For this review, take the finished solid that the model builds, in its own axes (mm). A direction names the side the tool comes from. Round coordinates to 2 decimals unless told otherwise and drop trailing zeros. Write each loop counter-clockwise with the first axis right and the second up, starting at its lowest first coordinate (ties: lowest second). Pieces come first, ordered by that corner, then holes. Notation, with made-up numbers: M 29.5,31 L 67.5,31 A30 ccw 67.5,63 Z; hole C 2,77.5 d11. An arc over 180 degrees is marked long. Use one line per item in the form item = value. Start each with the question number.
Item 1: Add section B-B (y = -8.25). State the section outline as (x, z) points.
Item 2: For faces 4 (the cylindrical face through (-19.274, 5.334, -19.435)), 5 (the flat face through (0, 0, 0)), list the 3-axis set-ups (+Z, -Z, +X, -X, +Y, -Y) from which the entire face can be reached by the end or side of a thin tool; tool diameter is ignored.
Item 3: For line 1 (Z direction, x = 17.5, y = 6.25) (3 decimals); line 2 (X direction, y = 6.25, z = -17.5) (3 decimals); line 3 (X direction, y = -8.25, z = -13), list the stretches that pass through material, from the lowest coordinate up. Write a range as [from, to].
Item 4: Add section A-A (z = 17.5). State the section outline as (x, y) points (3 decimals), and give its area (3 significant figures).
Item 5: Add section C-C (x = -17.5). State the section outline as (y, z) points (3 decimals), and give its area (3 significant figures).
Item 6: Draft analysis for pull direction Z (two halves, no side actions). For faces 1 (the flat face through (26, -12, 0)), 2 (the flat face through (0, 4, -25)), 3 (the cylindrical face through (15.726, 5.334, -19.435)), state which applies: released by +Z, released by -Z, zero draft, split by the parting line, or undercut.
Item 7: Add section D-D (y = 7.25). State the section outline as (x, z) points (3 decimals).
Item 8: For P1, Ø3, axis at x = -15.5, z = -2, coming from the -Y side, flat-tipped, find the tip position at first contact; note if it passes through.
Autodesk Inventor part; units mm, degrees
ref_plane "YZ Plane" through (0, 0, 0) normal (1, 0, 0) x (0, 1, 0)
ref_plane "XZ Plane" through (0, 0, 0) normal (0, 1, 0) x (-1, 0, 0)
ref_plane "XY Plane" through (0, 0, 0) normal (0, 0, 1) x (1, 0, 0)
sketch "Sketch1" plane through (0, 0, 0) normal (0, 1, 0) x (-1, 0, 0)
  line L0 (29, -25) -> (-29, -25)
  line L1 (-29, -25) -> (-29, 25)
  line L2 (-29, 25) -> (29, 25)
  line L3 (29, 25) -> (29, -25)
  line L4 (29, -25) -> (-29, 25) construction
  line L5 (-29, -25) -> (29, 25) construction
  point P0 (0, 0)
  dimension "d0" = 58
  dimension "d1" = 50
extrude "Extrusion1" add sketch "Sketch1" along normal blind 10.8204
sketch "Sketch2" plane through (0, 0, 0) normal (0, -1, 0) x (1, 0, 0)
  line L0 (-29, -25) -> (29, -25)
  line L1 (29, -25) -> (29, 25)
  line L2 (29, 25) -> (-29, 25)
  line L3 (-29, 25) -> (-29, -25)
  line L4 (-24, 25) -> (-24, -25)
  line L5 (24, 25) -> (24, -25)
  point P0 (0, 0)
  dimension "d4" = 5
  dimension "d5" = 5
extrude "Extrusion2" add sketch "Sketch2" along normal blind 12 contours L3 L2 L4 L0 | L5 L2 L1 L0
sketch "Sketch3" plane through (0, 10.8204, 0) normal (0, 1, 0) x (1, 0, 0)
  line L0 (29, 25) -> (-29, 25)
  line L1 (-29, 25) -> (-29, -25)
  point P0 (0, 0)
  point P1 (-17.5, 17.5)
  point P2 (17.5, 17.5)
  point P3 (-17.5, -17.5)
  point P4 (17.5, -17.5)
  dimension "d10" = 35
  dimension "d13" = 35
  dimension "d16" = 11.5
  dimension "d17" = 58
  dimension "d18" = 50
  dimension "d19" = 7.5
hole "Hole1" at (-17.5, 10.8204, -17.5) at (17.5, 10.8204, -17.5) at (-17.5, 10.8204, 17.5) at (17.5, 10.8204, 17.5) direction (0, -1, 0) diameter 5.25 end through all
equation "\"d5\" = d4"
properties part number "sbr20uu_standoff"
Calculated:
q1.outline = M -29,-25 L -24,-25 L -24,25 L -29,25 Z; M 24,-25 L 29,-25 L 29,25 L 24,25 Z
q2.face_4 = +Y, -Y
q2.face_5 = +Z, -Z, -Y
q3.line_1 = [-25, -20.125], [-14.875, 14.875], [20.125, 25]
q3.line_2 = [-29, -20.125], [-14.875, 14.875], [20.125, 29]
q3.line_3 = [-29, -24], [24, 29]
q4.outline = M -29,-12 L -24,-12 L -24,0 L -20.125,0 L -20.125,10.82 L -29,10.82 Z; M -14.875,0 L 14.875,0 L 14.875,10.82 L -14.875,10.82 Z; M 20.125,0 L 24,0 L 24,-12 L 29,-12 L 29,10.82 L 20.125,10.82 Z
q4.area = 634 mm^2
q5.outline = M 0,-25 L 10.82,-25 L 10.82,-20.125 L 0,-20.125 Z; M 0,-14.875 L 10.82,-14.875 L 10.82,14.875 L 0,14.875 Z; M 0,20.125 L 10.82,20.125 L 10.82,25 L 0,25 Z
q5.area = 427 mm^2
q6.face_1 = zero draft
q6.face_2 = released by -Z
q6.face_3 = undercut
q7.outline = M -29,-25 L 29,-25 L 29,25 L -29,25 Z; hole C -17.5,-17.5 d5.25; hole C -17.5,17.5 d5.25; hole C 17.5,-17.5 d5.25; hole C 17.5,17.5 d5.25
q8.P1 = 0
